from build123d import *

# Parameters (mm, degrees)
BOSS_EXTRUDE1_DEPTH = 12.5
BOSS_EXTRUDE2_DEPTH = 4.4
SKETCH3_R           = 2.5
BOSS_EXTRUDE3_DEPTH = 2.9
SKETCH4_R           = 1
CUT_EXTRUDE1_DEPTH  = 40.466061369


with BuildPart() as part:
    # Sketch1 → Boss-Extrude1 (new body)
    with BuildSketch(Plane(origin=(0, 0, 0), x_dir=(0, 0, -1), z_dir=(1, 0, 0))):
        Polygon((0, 0), (0, 5), (-15.8, 5), (-15.8, 27.6), (0, 27.6), (0, 32.6), (2.6, 32.6), (2.6, 27.6), (6.8, 27.6), (6.8, 5), (2.6, 5), (2.6, 0), align=None)
    extrude(amount=BOSS_EXTRUDE1_DEPTH)

    # Sketch2 → Boss-Extrude2 (add)
    with BuildSketch(Plane(origin=(0, 0, -6.8), x_dir=(-1, 0, 0), z_dir=(0, 0, -1))):
        with BuildLine():
            ThreePointArc((-8.910810534, 15.694685039), (-6.25, 27.6), (-3.589189466, 15.694685039))
            ThreePointArc((-3.589189466, 15.694685039), (-6.25, 12.25), (-8.910810534, 15.694685039))
        make_face()
    extrude(amount=BOSS_EXTRUDE2_DEPTH)

    # Sketch3 → Boss-Extrude3 (add)
    with BuildSketch(Plane(origin=(0, 0, -11.2), x_dir=(-1, 0, 0), z_dir=(0, 0, -1))):
        with Locations(Location((-6.25, 21.35, 0), (0, 0, 90))):
            Circle(SKETCH3_R)
    extrude(amount=BOSS_EXTRUDE3_DEPTH)

    # Sketch4 → Cut-Extrude1 (cut, through all)
    with BuildSketch(Plane(origin=(0, 0, -2.6), x_dir=(-1, 0, 0), z_dir=(0, 0, -1))):
        with Locations(Location((-6.25, 30.1, 0), (0, 0, 90))):
            Circle(SKETCH4_R)
        with Locations(Location((-6.25, 2.5, 0), (0, 0, 90))):
            Circle(SKETCH4_R)
    extrude(amount=-CUT_EXTRUDE1_DEPTH, mode=Mode.SUBTRACT)


solid = part.part
Read the model definition and answer for the solid it produces. Units are mm, in the model's axes. A direction names the side the tool comes from. Round coordinates to 2 decimals unless told otherwise and drop trailing zeros. Write each loop counter-clockwise with the first axis right and the second up, starting at its lowest first coordinate (ties: lowest second). Pieces come first, ordered by that corner, then holes. Notation, with made-up numbers: M -0.75,51 L 57.25,51 A10 ccw 57.25,59 Z; hole C 88,-12 d1. An arc over 180 degrees is marked long. Use a Markdown table: item, result.
1) The part is cut by section B-B (z = -1). Write down the section's boundary in (x, y).
Answers follow:
| item | result |
|---|---|
| outline | M 0,0 L 12.5,0 L 12.5,32.6 L 0,32.6 Z; hole C 6.25,2.5 d2; hole C 6.25,30.1 d2 |
2) For a pull along X with two mould halves and no side action, classify faces 4 (the flat face through (12.5, 17, 4)), 5 (the cylindrical face through (6.926, 1.763, -1.318)), 6 (the flat face through (6, 16, 15.8)) as pulls with the +X half, pulls with the -X half, needs draft (parallel to the pull), parting line crosses it, or undercut.
Answers follow:
| item | result |
|---|---|
| face 4 | pulls with the +X half |
| face 5 | undercut |
| face 6 | needs draft |
3) The part is cut by section A-A (y = 29.5). Write down the section's boundary in (x, z).
Answers follow:
| item | result |
|---|---|
| outline | M 0,-2.6 L 5.45,-2.6 L 5.45,0 L 0,0 Z; M 7.05,-2.6 L 12.5,-2.6 L 12.5,0 L 7.05,0 Z |
4) The part is cut by section D-D (x = 2.75). Write down the section's boundary in (y, z), plus the area to 3 significant figures.
Answers follow:
| item | result |
|---|---|
| outline | M 0,-2.6 L 5,-2.6 L 5,-6.8 L 16.17,-6.8 L 16.17,-11.2 L 26.53,-11.2 L 26.53,-6.8 L 27.6,-6.8 L 27.6,-2.6 L 32.6,-2.6 L 32.6,0 L 27.6,0 L 27.6,15.8 L 5,15.8 L 5,0 L 0,0 Z |
| area | 582 mm2 |
5) Flat-ended cylindrical pins translate along their axes: pin 1 (1.5 mm diameter, centred on x = 3.5, y = 3, fed in from -Z); pin 2 (7 mm diameter, centred on x = 9, y = 23, fed in from -Z); pin 3 (4 mm diameter, centred on x = 9, y = 1.5, fed in from +Z); pin 4 (3.5 mm diameter, centred on x = 5, z = -5.5, fed in from -Y). Find the tip coordinate at first contact, or state that the pin passes through.
Answers follow:
| item | result |
|---|---|
| pin 1 | stops at z = -2.6 |
| pin 2 | stops at z = -14.1 |
| pin 3 | stops at z = 0 |
| pin 4 | stops at y = 5 |
6) The part is cut by section C-C (y = 2.5). Write down the section's boundary in (x, z).
Answers follow:
| item | result |
|---|---|
| outline | M 0,-2.6 L 5.25,-2.6 L 5.25,0 L 0,0 Z; M 7.25,-2.6 L 12.5,-2.6 L 12.5,0 L 7.25,0 Z |
7) Straight lines are drawn through the part: line 1 along X through (y, z) = (2.5, -2); line 2 along Z through (x, y) = (1, 14.5); line 3 along Y through (x, z) = (10.5, 1.5). For each, find the intervals that lie inside material, in ascending order. Write a range as [from, to].
Answers follow:
| item | result |
|---|---|
| line 1 | x = [0, 5.25], [7.25, 12.5] |
| line 2 | z = [-6.8, 15.8] |
| line 3 | y = [5, 27.6] |
8) A tool of negligible diameter and unlimited length cuts with its end or side. For faces 1 (the flat face through (6, 5, -5)), 2 (the flat face through (6, 27.6, 8)), 3 (the flat face through (6, 4, 0)), from which of +Z, -Z, +X, -X, +Y, -Y can it reach the whole face along a straight path? Write none if from no direction.
Answers follow:
| item | result |
|---|---|
| face 1 | -Z, +X, -X, -Y |
| face 2 | +Z, +X, -X, +Y |
| face 3 | +Z, +X, -X, -Y |
